from build123d import *

# Parameters (mm, degrees)
F0_R     = 2.5
F0_W     = 8
F0_H     = 20
F0_H_2   = 5
F0_W_2   = 24
F1_DEPTH = 3
F2_DEPTH = 20
F3_DEPTH = 17
F4_R     = 2.99999


# Not quite as in the source:
# - a fillet or chamfer is up to 0.001 mm smaller than in the source, because OpenCascade refuses the exact size


with BuildPart() as f1:
    # F0 (on Top) → F1 (new body)
    with BuildSketch(Plane.XY):
        Polygon((-5.5937515758, 18.9813033898), (-45.5937515758, 18.9813033898), (-45.5937515758, -6.0186966102), (-37.5937515758, -6.0186966102), (-37.5937515758, -26.0186966102), (-13.5937515758, -26.0186966102), (-13.5937515758, -6.0186966102), (-5.5937515758, -6.0186966102), align=None)
        with Locations((-25.5937515758, -10.5820312165)):
            Circle(F0_R, mode=Mode.SUBTRACT)
        with Locations((-25.5937515758, 6.1523453332)):
            Circle(F0_R, mode=Mode.SUBTRACT)
        with Locations((-41.5937515758, -16.0186966102)):
            Rectangle(F0_W, F0_H)
        with Locations((-41.5937515758, -28.5186966102)):
            Rectangle(F0_W, F0_H_2)
        with Locations((-25.5937515758, -28.5186966102)):
            Rectangle(F0_W_2, F0_H_2)
        with Locations((-9.5937515758, -28.5186966102)):
            Rectangle(F0_W, F0_H_2)
        with Locations((-9.5937515758, -16.0186966102)):
            Rectangle(F0_W, F0_H)
    extrude(amount=-F1_DEPTH)

    # F0 (on Top) → F2 (join)
    with BuildSketch(Plane.XY):
        with Locations((-41.5937515758, -16.0186966102)):
            Rectangle(F0_W, F0_H)
        with Locations((-9.5937515758, -16.0186966102)):
            Rectangle(F0_W, F0_H)
        with Locations((-9.5937515758, -28.5186966102)):
            Rectangle(F0_W, F0_H_2)
        with Locations((-41.5937515758, -28.5186966102)):
            Rectangle(F0_W, F0_H_2)
    extrude(amount=F2_DEPTH)

    # F0 (on Top) → F3 (cut)
    with BuildSketch(Plane.XY):
        with Locations((-41.5937515758, -16.0186966102)):
            Rectangle(F0_W, F0_H)
        with Locations((-9.5937515758, -16.0186966102)):
            Rectangle(F0_W, F0_H)
    extrude(amount=F3_DEPTH, mode=Mode.SUBTRACT)

    # F4 (radius 3 in the source; OpenCascade refuses exactly that, so slightly less here)
    f4_edges = [f1.edges().sort_by_distance(p)[0] for p in [
        (-41.593752, -31.018697, 20),
        (-9.593752, -31.018697, 20),
        (-41.593752, -6.018697, 20),
        (-9.593752, -6.018697, 20),
        (-41.593752, -26.018697, 17),
        (-9.593752, -26.018697, 17),
        (-9.593752, -26.018697, 0),
        (-41.593752, -26.018697, 0),
    ]]
    fillet(f4_edges, radius=F4_R)


solid = f1.part
Design review of the part built by this model. Coordinates are the model's own, in mm. A direction names the side the tool comes from. Round coordinates to 2 decimals unless told otherwise and drop trailing zeros. Write each loop counter-clockwise with the first axis right and the second up, starting at its lowest first coordinate (ties: lowest second). Pieces come first, ordered by that corner, then holes. Notation, with made-up numbers: M -27,34.5 L 31,34.5 A20 ccw 31,58.5 Z; hole C 34,43.5 d4. An arc over 180 degrees is marked long. One line per item, written item: value. Start each with the question number.
1. Draft analysis for pull direction Z (two halves, no side actions). For faces 1 (the face through (-9.54, -30.12, 19.14)), 2 (the face through (-41.54, -25.12, 16.14)), 3 (the face through (-45.594, -13, -1)), state which applies: pulls with the +Z half, pulls with the -Z half, needs draft (parallel to the pull), parting line crosses it, or undercut.
2. Take a section at B-B on y = -21. State the section outline as (x, z) points, then the cut area to 3 significant figures.
3. Take a section at D-D on y = -10. State the section outline as (x, z) points.
4. Clearance check with flat-ended pins moving along their axes: P1, Ø4, axis at x = -10.5, y = -1, coming from the +Z side; P2, Ø9, axis at x = -9.5, z = 7, coming from the +Y side. State where each tip first meets the part, or that it passes through.
5. For faces 4 (the face through (-10, -14, 17)), 5 (the face through (-37.594, -27, 14)), 6 (the face through (-26, -6, -3)), list the 3-axis set-ups (+Z, -Z, +X, -X, +Y, -Y) from which the entire face can be reached by the end or side of a thin tool; tool diameter is ignored.
6. Take a section at A-A on z = 12.5. State the section outline as (x, y) points, then the cut area to 3 significant figures.
7. To check wall thickness, follow probe 1 along Z at (x, y) = (-11.5, -9); probe 2 along X at (y, z) = (-28, 12); probe 3 along Z at (x, y) = (-18, -12). State the ranges of each line that lie inside material, in increasing order. Write a range as from..to.
Computed:
1. face 1: pulls with the +Z half
1. face 2: undercut
1. face 3: needs draft
2. outline: M -45.59,-3 L -5.59,-3 L -5.59,0 L -45.59,0 Z; M -45.59,17 L -37.59,17 L -37.59,20 L -45.59,20 Z; M -13.59,17 L -5.59,17 L -5.59,20 L -13.59,20 Z
2. area: 168 mm²
3. outline: M -45.59,-3 L -28.03,-3 L -28.03,0 L -45.59,0 Z; M -45.59,17 L -37.59,17 L -37.59,20 L -45.59,20 Z; M -23.16,-3 L -5.59,-3 L -5.59,0 L -23.16,0 Z; M -13.59,17 L -5.59,17 L -5.59,20 L -13.59,20 Z
4. P1: stops at z = 0
4. P2: stops at y = -25.98
5. face 4: +X, -X, +Y
5. face 5: +Z, +Y, -Y
5. face 6: -Z, +X, -X, +Y, -Y
6. outline: M -45.59,-31.02 L -37.59,-31.02 L -37.59,-26.02 L -45.59,-26.02 Z; M -13.59,-31.02 L -5.59,-31.02 L -5.59,-26.02 L -13.59,-26.02 Z
6. area: 80.0 mm²
7. probe 1: z = -3..0, 17..20
7. probe 2: x = -45.59..-37.59, -13.59..-5.59
7. probe 3: z = -3..0
